Here's how the part is built. I have some questions about the finished solid (model axes, mm). A direction names the side the tool comes from. Give positions to 0.01 mm unless a question says otherwise; leave off trailing zeros. Loops run counter-clockwise (first coordinate to the right, second up) from the corner with the lowest first, then second, coordinate; pieces in that order, holes last. Notation, with made-up numbers: (24.25, 65) - (69.25, 65) arc R15 ccw to (69.25, 78) - close; hole circle Ø2 at (11.25, -10.75). An arc over 180 degrees is marked (long way). Return JSON: item names as keys, results as strings. Group by question number.
(1) If we section it at A-A (y = 20): Please give me the cut outline in (x, z), then the cut area to 3 significant figures.
(2) For P1, Ø8, axis at x = 119.5, y = 122, coming from the +Z side; P2, Ø1, axis at x = 87, y = 119.5, coming from the -Z side; P3, Ø1.5, axis at x = 278.5, z = -40.5, coming from the -Y side; P4, Ø6, axis at y = 148, z = -60, coming from the +X side, each with a flat end and sliding along its axis, tell me the tip position at first contact or that it passes through.
(3) I need wall thicknesses on probe 1 along Z at (x, y) = (-5, 148); probe 2 along X at (y, z) = (133.5, 42); probe 3 along Y at (x, z) = (115, 53). Which ranges of each line are inside material? Lowest first, please. Write a range as [from, to].
(4) If we mould it in two halves opening along Z, with no side actions, what happens to faces 1 (the cylindrical face through (2.46, 134.99, 12.15)), 2 (the flat face through (-16, 153, -58)), 3 (the flat face through (277.465, 44.044, 65.061))? For each: released by +Z, released by -Z, zero draft, split by the parting line, or undercut.
(5) If we section it at B-B (x = 35): Please give me the cut outline in (y, z).
(6) On a 3-axis mill with a long thin cutter (end or side, diameter ignored), from which of +Z, -Z, +X, -X, +Y, -Y can I reach the whole of each face in a straight line? I mean faces 4 (the flat face through (138, 0, 80)), 5 (the cylindrical face through (277.46, 134.99, 12.15)), 6 (the flat face through (2.465, 44.044, 65.061)). Say none if no direction works.
```python
from build123d import *
from build123d.topology import SkipClean

# Parameters (mm, degrees)
BOSS_EXTRUDE1_DEPTH     = 3
BOSS_EXTRUDE2_DEPTH     = 280
CUT_EXTRUDE2_DEPTH      = 385.010416525
CUT_EXTRUDE2_DEPTH_BACK = 385.010416525
SKETCH3_W               = 270
SKETCH3_H               = 200
CUT_EXTRUDE3_DEPTH      = 385.010416525
CUT_EXTRUDE3_DEPTH_BACK = 385.010416525
SKETCH4_R               = 5
BOSS_EXTRUDE3_START     = 16
SKETCH5_R               = 10
SKETCH5_R_2             = 5
BOSS_EXTRUDE3_DEPTH     = 16
SKETCH6_R               = 10
SKETCH6_R_2             = 5
BOSS_EXTRUDE4_DEPTH     = 16
BOSS_EXTRUDE5_DEPTH     = 270


with BuildPart() as part:
    # Sketch1 → Boss-Extrude1 (new body)
    with BuildSketch(Plane(origin=(0, 0, 0), x_dir=(1, 0, 0), z_dir=(0, 1, 0))):
        Polygon((0, 0), (280, 0), (280, -100), (230, -100), (230, -210), (50, -210), (50, -100), (0, -100), align=None)
    extrude(amount=BOSS_EXTRUDE1_DEPTH)

    # Sketch2 → Boss-Extrude2 (add, through all)
    with BuildSketch(Plane.ZY):
        with BuildLine():
            Line((15, 0), (15, 3))
            Line((15, 3), (15, 128))
            ThreePointArc((15, 128), (12.071067812, 135.071067812), (5, 138))
            Line((5, 138), (-60, 138))
            ThreePointArc((-60, 138), (-70, 148), (-60, 158))
            Line((-60, 158), (34.580462925, 158))
            ThreePointArc((34.580462925, 158), (46.051991652, 154.383040886), (53.37431534, 144.840402867))
            Line((53.37431534, 144.840402867), (105, 3))
            Line((105, 3), (105, 0))
            Line((105, 0), (80, 0))
            Line((80, 0), (80, 3))
            Line((80, 3), (49.698463104, 86.252788397))
            ThreePointArc((49.698463104, 86.252788397), (44.131759112, 89.466726445), (40, 84.54268768))
            Line((40, 84.54268768), (40, 3))
            Line((40, 3), (40, 0))
            Line((40, 0), (15, 0))
        make_face()
    extrude(amount=-BOSS_EXTRUDE2_DEPTH)

    # Sketch3 → Cut-Extrude2 (cut, two sides: drawn at the far end of the back side and taken through both)
    with BuildSketch(Plane(origin=(0, 0, 0), x_dir=(-1, 0, 0), z_dir=(0, 0, -1)).offset(-CUT_EXTRUDE2_DEPTH_BACK)):
        with Locations((-140, 103)):
            Rectangle(SKETCH3_W, SKETCH3_H)
    extrude(amount=CUT_EXTRUDE2_DEPTH + CUT_EXTRUDE2_DEPTH_BACK, mode=Mode.SUBTRACT)

    # Sketch4 → Cut-Extrude3 (cut, two sides: drawn at the far end of the back side and taken through both)
    with BuildSketch(Plane.ZY.offset(-CUT_EXTRUDE3_DEPTH_BACK)):
        with Locations((-60, 148)):
            Circle(SKETCH4_R)
    extrude(amount=CUT_EXTRUDE3_DEPTH + CUT_EXTRUDE3_DEPTH_BACK, mode=Mode.SUBTRACT)

    # Sketch5 → Boss-Extrude3 (add)
    with SkipClean():  # the faces are left unmerged after this step: merging them gives an invalid solid
        with BuildSketch(Plane.ZY.offset(BOSS_EXTRUDE3_START)):
            with Locations((-60, 148)):
                Circle(SKETCH5_R)
            with Locations((-60, 148)):
                Circle(SKETCH5_R_2, mode=Mode.SUBTRACT)
        extrude(amount=-BOSS_EXTRUDE3_DEPTH)

    # Sketch6 → Boss-Extrude4 (add)
    with SkipClean():  # the faces are left unmerged after this step: merging them gives an invalid solid
        with BuildSketch(Plane(origin=(280, 0, 0), x_dir=(0, 0, -1), z_dir=(1, 0, 0))):
            with Locations(Location((60, 148, 0), (0, 0, 90))):
                Circle(SKETCH6_R)
            with Locations((60, 148)):
                Circle(SKETCH6_R_2, mode=Mode.SUBTRACT)
        extrude(amount=BOSS_EXTRUDE4_DEPTH)

    # Sketch7 → Boss-Extrude5 (add)
    with SkipClean():  # the faces are left unmerged after this step: merging them gives an invalid solid
        with BuildSketch(Plane(origin=(5, 0, 0), x_dir=(0, 0, -1), z_dir=(1, 0, 0))):
            Polygon((0, 0), (-3, 0), (36.02381866, 145.638873943), (38.822856765, 144.888873943), align=None)
        extrude(amount=BOSS_EXTRUDE5_DEPTH)


solid = part.part
```
Values:
{
 "1": {"outline": "(0, 15) - (5, 15) - (5, 40) - (0, 40) - close; (0, 73.81) - (5, 73.81) - (5, 98.81) - (0, 98.81) - close; (5, -5.36) - (275, -5.36) - (275, -2.36) - (5, -2.36) - close; (275, 15) - (280, 15) - (280, 40) - (275, 40) - close; (275, 73.81) - (280, 73.81) - (280, 98.81) - (275, 98.81) - close", "area": "1,310 mm2"},
 "2": {"P1": "z = -28.62", "P2": "z = -32.15", "P3": "y = 138", "P4": "through"},
 "3": {"probe 1": "[-70, -65], [-55, -50]", "probe 2": "[0, 5], [275, 280]", "probe 3": "[0, 3]"},
 "4": {"face 1": "released by -Z", "face 2": "zero draft", "face 3": "undercut"},
 "5": {"outline": "(0, 0) - (144.89, -38.82) - (145.64, -36.02) - (3, 2.2) - (3, 105) - (0, 105) - close"},
 "6": {"face 4": "+Z, -Z, +X, -X, -Y", "face 5": "-Z, +X, -X", "face 6": "+X, -X"}
}
